```python
from build123d import *

# Parameters (mm, degrees)
SKETCH1_W           = 78
SKETCH1_H           = 24
BOSS_EXTRUDE1_DEPTH = 5
SKETCH2_W           = 78
SKETCH2_H           = 8
BOSS_EXTRUDE2_DEPTH = 27.5
FILLET1_R           = 20
SKETCH3_W           = 67
SKETCH3_H           = 19.595917942
CUT_EXTRUDE1_DEPTH  = 16
SKETCH4_W           = 33.86
SKETCH4_H           = 9.88
SKETCH4_R           = 2.75
BOSS_EXTRUDE3_DEPTH = 78
FILLET2_R           = 20
SKETCH5_W           = 68
SKETCH5_H           = 20
CUT_EXTRUDE2_DEPTH  = 34
SKETCH6_W           = 68
SKETCH6_H           = 9.88
CUT_EXTRUDE3_DEPTH  = 34


with BuildPart() as part:
    # Sketch1 → Boss-Extrude1 (new body)
    with BuildSketch(Plane(origin=(0, 0, 0), x_dir=(1, 0, 0), z_dir=(0, 1, 0))):
        Rectangle(SKETCH1_W, SKETCH1_H)
    extrude(amount=BOSS_EXTRUDE1_DEPTH)

    # Sketch2 → Boss-Extrude2 (add)
    with BuildSketch(Plane(origin=(0, 5, 0), x_dir=(1, 0, 0), z_dir=(0, 1, 0))):
        with Locations((0, -8)):
            Rectangle(SKETCH2_W, SKETCH2_H)
    extrude(amount=BOSS_EXTRUDE2_DEPTH)

    # Fillet1
    # the kernel refuses this fillet: 20 mm, written as the material it adds along each edge
    with BuildSketch(Plane(origin=(39, 5, 4), x_dir=(0, 0, -1), z_dir=(-1, 0, 0))) as fillet1_piece_1:
        with BuildLine():
            CenterArc((20, -19.595917942), FILLET1_R, 101.536959033, 78.463040967)
            Line((0, -19.595917942), (-0.4, -19.595917942))
            Line((-0.4, -19.595917942), (-0.4, 0))
            Line((-0.4, 0), (0, 0.4))
            ThreePointArc((0, 0.4), (8, 0.4), (15.92, 0.391918359))
            Line((15.92, 0.391918359), (16, 0))
        make_face()
    extrude(amount=78)

    # Sketch3 → Cut-Extrude1 (cut)
    with BuildSketch(Plane(origin=(0, 0, -12), x_dir=(-1, 0, 0), z_dir=(0, 0, -1))):
        with Locations((0, 14.797958971)):
            Rectangle(SKETCH3_W, SKETCH3_H)
    extrude(amount=-CUT_EXTRUDE1_DEPTH, mode=Mode.SUBTRACT)

    # Sketch4 → Boss-Extrude3 (add)
    with BuildSketch(Plane.ZY.offset(39)):
        with Locations((28.93, 27.56)):
            Rectangle(SKETCH4_W, SKETCH4_H)
        with Locations((38.86, 27.56)):
            Circle(SKETCH4_R, mode=Mode.SUBTRACT)
    extrude(amount=-BOSS_EXTRUDE3_DEPTH)

    # Fillet2
    fillet2_edges = [part.edges().sort_by_distance(p)[0] for p in [
        (0, 22.62, 12),
    ]]
    fillet(fillet2_edges, radius=FILLET2_R)

    # Sketch5 → Cut-Extrude2 (cut)
    with BuildSketch(Plane.XY.offset(45.86)):
        with Locations((0, 12.62)):
            Rectangle(SKETCH5_W, SKETCH5_H)
    extrude(amount=-CUT_EXTRUDE2_DEPTH, mode=Mode.SUBTRACT)

    # Sketch6 → Cut-Extrude3 (cut)
    with BuildSketch(Plane.XY.offset(45.86)):
        with Locations((0, 27.56)):
            Rectangle(SKETCH6_W, SKETCH6_H)
    extrude(amount=-CUT_EXTRUDE3_DEPTH, mode=Mode.SUBTRACT)


solid = part.part
```
Could you check a few things on this model? Use its own coordinates, in mm. A direction names the side the tool comes from. Coordinates: 2 decimals unless noted, no trailing zeros. Loops run counter-clockwise (first coordinate to the right, second up) from the corner with the lowest first, then second, coordinate; pieces in that order, holes last.
1) Imagine slicing it at B-B (z = 38.86). List the corners of the cut face in (x, y) for me.
Reported:
outline: (-39, 22.62) - (-34, 22.62) - (-34, 24.81) - (-39, 24.81) - close; (-39, 30.31) - (-34, 30.31) - (-34, 32.5) - (-39, 32.5) - close; (34, 22.62) - (39, 22.62) - (39, 24.81) - (34, 24.81) - close; (34, 30.31) - (39, 30.31) - (39, 32.5) - (34, 32.5) - close
2) Will these pins go through, and if not, where does the flat tip stop? pin 1 Ø1.3 at (x, y) = (-3, 2) entering from +Z; pin 2 Ø8 at (x, y) = (2, 12.5) entering from -Z; pin 3 Ø8 at (y, z) = (15, -5) entering from -X; pin 4 Ø12 at (x, y) = (13.5, 5.5) entering from -Z.
Reported:
pin 1: stops at z = 12
pin 2: stops at z = 4
pin 3: passes through
pin 4: stops at z = -12
3) Imagine slicing it at D-D (x = 29). List the corners of the cut face in (y, z) for me.
Reported:
outline: (0, -12) - (5, -12) - (5, 4) - (32.5, 4) - (32.5, 11.86) - (2.62, 11.86) - (2.62, 12) - (0, 12) - close
4) Thinking about a two-plate mould opening in Y: for faces 1 (the face through (-36.53, 25.12, 40.13)), 2 (the face through (36.535, 16.917, 18.014)), 3 (the face through (-37, 27, 45.86)), which applies, released by +Y, released by -Y, zero draft, split by the parting line, or undercut?
Reported:
face 1: undercut
face 2: released by -Y
face 3: zero draft
5) Imagine slicing it at C-C (z = 18). List the corners of the cut face in (x, y) for me.
Reported:
outline: (-39, 16.9) - (-34, 16.9) - (-34, 32.5) - (-39, 32.5) - close; (34, 16.9) - (39, 16.9) - (39, 32.5) - (34, 32.5) - close
6) Which directions (+Z, -Z, +X, -X, +Y, -Y) give clear straight access to the entire face, cutting with the end or side of a thin tool? Please do faces 4 (the face through (36.47, 25.12, 40.13)), 5 (the face through (0, 18, 11.86)), 6 (the face through (39, 20, 17)), 7 (the face through (-1, 19, 4)), 8 (the face through (36, 22.62, 39)).
Reported:
face 4: +X, -X
face 5: +Z, +Y
face 6: +Z, -Z, +X, +Y, -Y
face 7: -Z, +Y
face 8: +Z, +X, -X, -Y
7) Imagine slicing it at A-A (y = 27.56). List the corners of the cut face in (x, z) for me.
Reported:
outline: (-39, 4) - (39, 4) - (39, 36.11) - (34, 36.11) - (34, 11.86) - (-34, 11.86) - (-34, 36.11) - (-39, 36.11) - close; (-39, 41.61) - (-34, 41.61) - (-34, 45.86) - (-39, 45.86) - close; (34, 41.61) - (39, 41.61) - (39, 45.86) - (34, 45.86) - close
8) Please list where these lines run through material, in increasing order: line 1 along Y through (x, z) = (-37.8, 38.86); line 2 along X through (y, z) = (7, 2); line 3 along Z through (x, y) = (29, 16.5).
Reported:
line 1: y = 22.62 to 24.81, 30.31 to 32.5
line 2: x = -39 to -33.5, 33.5 to 39
line 3: z = 4 to 11.86
